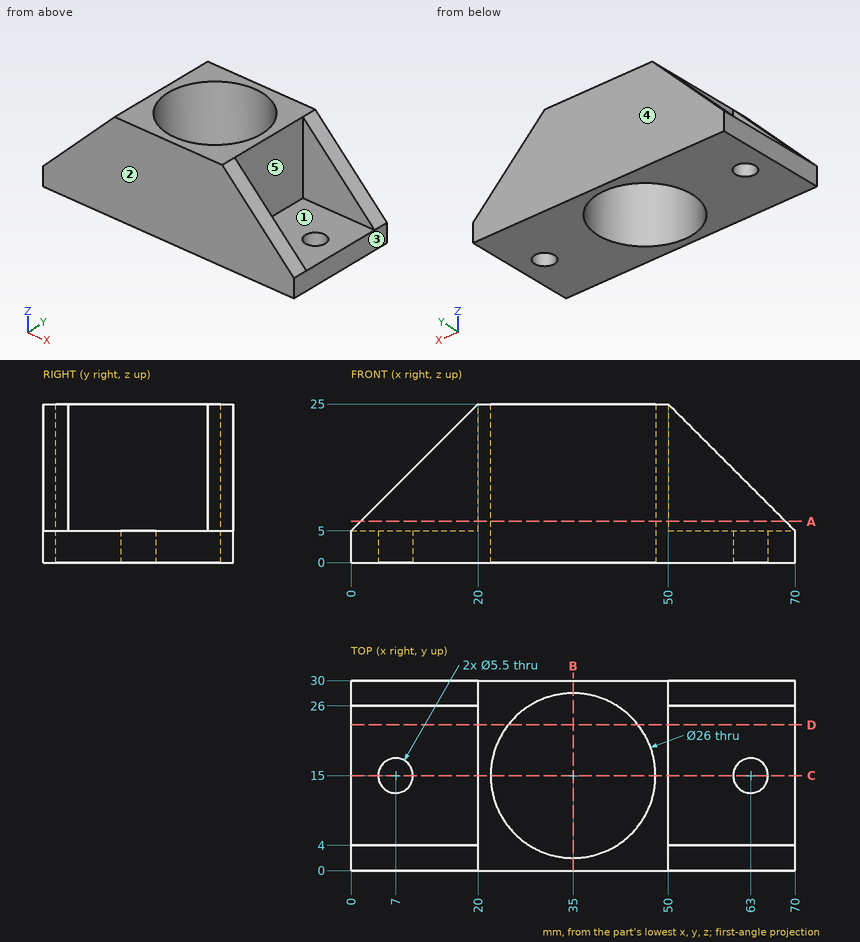
Geometry: see drawing. Coordinates: mm, zero at the bounding-box minimum. A direction names the side the tool comes from. Give positions to 0.01 mm unless a question says otherwise; leave off trailing zeros. Write each loop counter-clockwise with the first axis right and the second up, starting at its lowest first coordinate (ties: lowest second). Pieces come first, ordered by that corner, then holes. Notation, with made-up numbers: M 75.25,-14.5 L 108.25,-14.5 A18 cw 108.25,14.5 Z; hole C -24,-9.5 d5. An arc over 180 degrees is marked long. Answer in a Markdown table with one row per item. Add a question column.
(1) Section D-D on y = 23. Return loops of the section in (x, z).
(2) Section C-C on y = 15. Return loops of the section in (x, z).
(3) Ray query, line 1 (Y direction, x = 63, z = 1.55); line 2 (Y direction, x = 18, z = 11.25); line 3 (X direction, y = 16.25, z = 2.5). Return the intervals inside material, ascending.
(4) First-contact query: pin 1 (3 mm diameter, centred on y = 13.5, z = 8, fed in from +X); pin 2 (6 mm diameter, centred on x = 14.5, y = 16.5, fed in from +Z); pin 3 (1 mm diameter, centred on x = 13.5, z = 20.5, fed in from +Y). Flat tips, straight axial feed; report the tip coordinate or a pass-through.
(5) Section B-B on x = 35. Return loops of the section in (y, z).
(6) Section A-A on z = 6.5. Return loops of the section in (x, y).
(7) Reachability of the marked faces 1 and 2 from +Z, -Z, +X, -X, +Y, -Y: full face, straight path, thin tool, end or side. Return the list, or none.
(8) Mould query, pull axis Y, two halves, no side actions, for the marked faces 3, 4 and 5. Classes: +Y half, -Y half, draft (parallel to the pull), parting line (faces both ways), or undercut.
Result set:
| question | item | result |
|---|---|---|
| 1 | outline | M 0,0 L 24.75,0 L 24.75,25 L 20,25 L 20,5 L 0,5 Z; M 45.25,0 L 70,0 L 70,5 L 50,5 L 50,25 L 45.25,25 Z |
| 2 | outline | M 0,0 L 4.25,0 L 4.25,5 L 0,5 Z; M 9.75,0 L 22,0 L 22,25 L 20,25 L 20,5 L 9.75,5 Z; M 48,0 L 60.25,0 L 60.25,5 L 50,5 L 50,25 L 48,25 Z; M 65.75,0 L 70,0 L 70,5 L 65.75,5 Z |
| 3 | line 1 | y = 0 to 12.25, 17.75 to 30 |
| 3 | line 2 | y = 0 to 4, 26 to 30 |
| 3 | line 3 | x = 0 to 4.55, 9.45 to 22.06, 47.94 to 60.55, 65.45 to 70 |
| 4 | pin 1 | stops at x = 50 |
| 4 | pin 2 | stops at z = 5 |
| 4 | pin 3 | passes through |
| 5 | outline | M 0,0 L 2,0 L 2,25 L 0,25 Z; M 28,0 L 30,0 L 30,25 L 28,25 Z |
| 6 | outline | M 1.5,0 L 68.5,0 L 68.5,4 L 50,4 L 50,26 L 68.5,26 L 68.5,30 L 1.5,30 L 1.5,26 L 20,26 L 20,4 L 1.5,4 Z; hole C 35,15 d26 |
| 7 | face 1 | +Z, +X |
| 7 | face 2 | +Z, -Z, +X, -X, -Y |
| 8 | face 3 | draft |
| 8 | face 4 | +Y half |
| 8 | face 5 | undercut |
